Work out the finished part from the listing and answer in its coordinate system (mm). A direction names the side the tool comes from. Give positions to 0.01 mm unless a question says otherwise; leave off trailing zeros. Loops run counter-clockwise (first coordinate to the right, second up) from the corner with the lowest first, then second, coordinate; pieces in that order, holes last. Notation, with made-up numbers: M -31,65 L 17,65 A19 cw 17,75 Z; hole C 84.5,75.25 d7. An arc over 180 degrees is marked long. Write item = value, one per line. Start each with the question number.
1. Section A-A on y = -5.25 is taken. Determine the outline of the cut face in (x, z).
2. For faces 5 (the face through (-1.107, -3.131, 13.08)), 6 (the face through (-10.775, -3.131, -7.499)), determine the directions among +Z, -Z, +X, -X, +Y, -Y from which every point of the face is accessible in a straight line to the end or side of a thin tool.
3. Section B-B on z = -2 is taken. Determine the outline of the cut face in (x, y).
4. The mould has two halves that part along X. Classify faces 1 (the face through (-5, 0, 3)), 2 (the face through (10.567, -3.131, -7.486)), 3 (the face through (1.2, -3.1, 12.9)), 4 (the face through (-0.14, -3.131, -7.435)): released by +X, released by -X, zero draft, split by the parting line, or undercut.
5. Section D-D on z = 3.5 is taken. Determine the outline of the cut face in (x, y).
6. Consider L1, parallel to X at y = -1, z = 1.5; L2, parallel to X at y = -3.75, z = 3.5; L3, parallel to Z at x = 10, y = -2. Determine where each line is inside the solid, lowest interval first. Write a range as [from, to].
7. Flat-ended cylindrical pins translate along their axes: pin 1 Ø1.5 at (x, y) = (-9, -3) entering from +Z; pin 2 Ø1.5 at (y, z) = (-2, 14.5) entering from -X; pin 3 Ø1.5 at (x, y) = (-5.5, -4) entering from -Z. Find the tip coordinate at first contact, or state that the pin passes through.
8. Section C-C on x = -8 is taken. Determine the outline of the cut face in (y, z).
```python
from build123d import *

# Parameters (mm, degrees)
F1_DEPTH = 6.35


with BuildPart() as f1:
    # F0 (on Front) → F1 (new body)
    with BuildSketch(Plane.XZ):
        with BuildLine():
            ThreePointArc((-5.5879735466, 0.0171942529), (-4.7955253497, 2.8685676949), (-2.6580116206, 4.9153553508))
            Line((-2.6580116206, 4.9153553508), (-2.2450949747, 7.0888402589))
            ThreePointArc((-2.2450949747, 7.0888402589), (-6.4075834438, 3.7729275201), (-7.2879952633, -1.4755448838))
            Line((-7.2879952633, -1.4755448838), (-5.5879735466, 0.0171942529))
        make_face()
        with BuildLine():
            ThreePointArc((-2.6580116206, 4.9153553508), (0.0864898214, 5.5873306248), (2.8088774331, 4.8307299206))
            Line((2.8088774331, 4.8307299206), (2.3661382778, 7.0493614826))
            ThreePointArc((2.3661382778, 7.0493614826), (0.0636593572, 7.4355937993), (-2.2450949747, 7.0888402589))
            Line((-2.2450949747, 7.0888402589), (-2.6580116206, 4.9153553508))
        make_face()
        with BuildLine():
            Line((2.3661382778, 7.0493614826), (2.8088774331, 4.8307299206))
            ThreePointArc((2.8088774331, 4.8307299206), (4.8436427973, 2.7865513546), (5.588, 0))
            ThreePointArc((5.588, 0), (5.5874570768, -0.0778936122), (5.5858284127, -0.1557720884))
            Line((5.5858284127, -0.1557720884), (7.2616632349, -1.6001108475))
            ThreePointArc((7.2616632349, -1.6001108475), (7.3921872476, -0.8047828019), (7.435866302, 0))
            ThreePointArc((7.435866302, 0), (6.0368201707, 4.3415331264), (2.3661382778, 7.0493614826))
        make_face()
        with BuildLine():
            ThreePointArc((-2.2450949747, 7.0888402589), (0.0636593572, 7.4355937993), (2.3661382778, 7.0493614826))
            Line((2.3661382778, 7.0493614826), (0, 18.9064312726))
            Line((0, 18.9064312726), (-2.2450949747, 7.0888402589))
        make_face()
        with BuildLine():
            Line((16.373449777, -9.4532156363), (7.2616632349, -1.6001108475))
            ThreePointArc((7.2616632349, -1.6001108475), (6.4075834438, -3.7729275201), (4.9218569854, -5.5738165987))
            Line((4.9218569854, -5.5738165987), (16.373449777, -9.4532156363))
        make_face()
        with BuildLine():
            Line((7.2616632349, -1.6001108475), (5.5858284127, -0.1557720884))
            ThreePointArc((5.5858284127, -0.1557720884), (4.7955253497, -2.8685676949), (2.7790961135, -4.8479241735))
            Line((2.7790961135, -4.8479241735), (4.9218569854, -5.5738165987))
            ThreePointArc((4.9218569854, -5.5738165987), (6.4075834438, -3.7729275201), (7.2616632349, -1.6001108475))
        make_face()
        with BuildLine():
            ThreePointArc((2.7790961135, -4.8479241735), (-0.0864898214, -5.5873306248), (-2.9278167921, -4.7595832624))
            Line((-2.9278167921, -4.7595832624), (-5.0165682602, -5.4887294114))
            ThreePointArc((-5.0165682602, -5.4887294114), (-0.0636593572, -7.4355937993), (4.9218569854, -5.5738165987))
            Line((4.9218569854, -5.5738165987), (2.7790961135, -4.8479241735))
        make_face()
        with BuildLine():
            Line((-16.373449777, -9.4532156363), (-5.0165682602, -5.4887294114))
            ThreePointArc((-5.0165682602, -5.4887294114), (-6.471242801, -3.6626662791), (-7.2879952633, -1.4755448838))
            Line((-7.2879952633, -1.4755448838), (-16.373449777, -9.4532156363))
        make_face()
        with BuildLine():
            Line((-5.0165682602, -5.4887294114), (-2.9278167921, -4.7595832624))
            ThreePointArc((-2.9278167921, -4.7595832624), (-4.8820151711, -2.7187629299), (-5.5879735466, 0.0171942529))
            Line((-5.5879735466, 0.0171942529), (-7.2879952633, -1.4755448838))
            ThreePointArc((-7.2879952633, -1.4755448838), (-6.471242801, -3.6626662791), (-5.0165682602, -5.4887294114))
        make_face()
    extrude(amount=F1_DEPTH)


solid = f1.part
```
Verdict:
q1.outline = M -16.37,-9.45 L -5.02,-5.49 A7.44 ccw 4.92,-5.57 L 16.37,-9.45 L 7.26,-1.6 A7.44 ccw 2.37,7.05 L 0,18.91 L -2.25,7.09 A7.44 ccw -7.29,-1.48 Z; hole C 0,0 d11.18
q2.face_5 = +Z, -X, +Y, -Y
q2.face_6 = -Z, +Y, -Y
q3.outline = M -7.89,-6.35 L -5.22,-6.35 L -5.22,0 L -7.89,0 Z; M 5.22,-6.35 L 7.73,-6.35 L 7.73,0 L 5.22,0 Z
q4.face_1 = zero draft
q4.face_2 = undercut
q4.face_3 = released by +X
q4.face_4 = undercut
q5.outline = M -6.56,-6.35 L -4.36,-6.35 L -4.36,0 L -6.56,0 Z; M 4.36,-6.35 L 6.56,-6.35 L 6.56,0 L 4.36,0 Z
q6.L1 = [-7.28, -5.38], [5.38, 7.28]
q6.L2 = [-6.56, -4.36], [4.36, 6.56]
q6.L3 = [-7.29, -3.96]
q7.pin_1 = -2.32
q7.pin_2 = -0.98
q7.pin_3 = -5.92
q8.outline = M -6.35,-6.53 L 0,-6.53 L 0,-2.1 L -6.35,-2.1 Z
